Autodesk Inventor part; units mm, degrees
ref_plane "YZ Plane" through (0, 0, 0) normal (1, 0, 0) x (0, 1, 0)
ref_plane "XZ Plane" through (0, 0, 0) normal (0, 1, 0) x (-1, 0, 0)
ref_plane "XY Plane" through (0, 0, 0) normal (0, 0, 1) x (1, 0, 0)
sketch "Sketch1" plane through (0, 0, 0) normal (0, 1, 0) x (-1, 0, 0)
  line L0 (0, 0) -> (73.025, 0)
  line L1 (0, 0) -> (0, 73.025)
  line L2 (0, 73.025) -> (73.025, 0)
  line L3 (12.7, 0) -> (12.7, 60.325) construction
  line L4 (0, 12.7) -> (60.325, 12.7) construction
  circle A0 centre (12.7, 34.925) radius 3.302
  circle A1 centre (34.925, 12.7) radius 3.302
  circle A2 centre (50.8, 12.7) radius 3.302
  circle A3 centre (12.7, 50.8) radius 3.302
  circle A4 centre (12.7, 12.7) radius 3.302
  line L5 (0, 34.925) -> (38.1, 34.925) construction
  line L6 (34.925, 38.1) -> (34.925, 0) construction
  dimension "d0" = 73.025
  dimension "d1" = 73.025
  dimension "d2" = 12.7
  dimension "d3" = 12.7
  dimension "d4" = 6.604
  dimension "d5" = 6.604
  dimension "d6" = 6.604
  dimension "d7" = 6.604
  dimension "d8" = 15.875
  dimension "d9" = 15.875
  dimension "d10" = 6.604
  dimension "d14" = 34.925
  dimension "d15" = 34.925
extrude "Extrusion1" add sketch "Sketch1" along normal blind 3.175
fillet "Fillet1" radius 6.35 2 edges at (0, 1.5875, 73.025) (-73.025, 1.5875, 0)
equation "\"d0\" = d1"
equation "\"d2\" = d3"
equation "\"d4\" = d7"
equation "\"d5\" = d7"
equation "\"d6\" = d7"
equation "\"d9\" = d8"
equation "\"d10\" = d7"
equation "\"d15\" = d14"
properties part number "Chassis Corner Plate V1.500" material "Aluminum 6061"
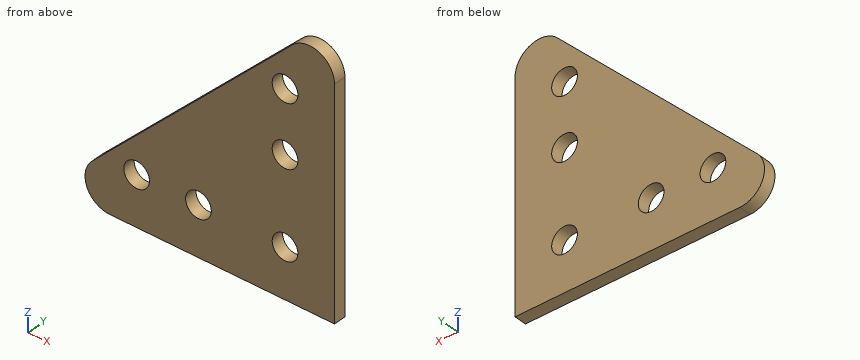
Could you check a few things on this model? Use its own coordinates, in mm. Coordinates: 2 decimals unless noted, no trailing zeros. Order: outer loops, then holes, each group sorted by start corner. A loop starts at its lowest first (then second) coordinate and runs counter-clockwise, first axis right, second up.
Q1. Suppose I cut it at A-A on z = 50.8. Please give me the cut outline in (x, y) (3 decimals).
Q2. Suppose I cut it at B-B on x = -12.7. Please give me the cut outline in (y, z) (3 decimals).
Q3. Suppose I cut it at C-C on y = 2.4. Please give me the cut outline in (x, z) (3 decimals), and give its area (3 significant figures).
Q4. Please list where these lines run through material, in increasing order: L1, parallel to Z at x = -12.7, y = 2.4 (3 decimals); L2, parallel to Z at x = -50.8, y = 1.3 (3 decimals); L3, parallel to X at y = 2.7, z = 11 (3 decimals).
Q5. Suppose I cut it at D-D on z = 12.7. Please give me the cut outline in (x, y) (3 decimals).
Answer:
1. outline: (-22.225, 0) - (-16.002, 0) - (-16.002, 3.175) - (-22.225, 3.175) - close; (-9.398, 0) - (0, 0) - (0, 3.175) - (-9.398, 3.175) - close
2. outline: (0, 0) - (3.175, 0) - (3.175, 9.398) - (0, 9.398) - close; (0, 16.002) - (3.175, 16.002) - (3.175, 31.623) - (0, 31.623) - close; (0, 38.227) - (3.175, 38.227) - (3.175, 47.498) - (0, 47.498) - close; (0, 54.102) - (3.175, 54.102) - (3.175, 60.325) - (0, 60.325) - close
3. outline: (-62.185, 10.84) arc R6.35 ccw to (-57.695, 0) - (0, 0) - (0, 57.695) arc R6.35 ccw to (-10.84, 62.185) - close; hole circle Ø6.604 at (-50.8, 12.7); hole circle Ø6.604 at (-34.925, 12.7); hole circle Ø6.604 at (-12.7, 12.7); hole circle Ø6.604 at (-12.7, 34.925); hole circle Ø6.604 at (-12.7, 50.8)
3. area: 2,400 mm2
4. L1: z = 0 to 9.398, 16.002 to 31.623, 38.227 to 47.498, 54.102 to 60.325
4. L2: z = 0 to 9.398, 16.002 to 22.225
4. L3: x = -62.025 to -53.631, -47.969 to -37.756, -32.094 to -15.531, -9.869 to 0
5. outline: (-60.325, 0) - (-54.102, 0) - (-54.102, 3.175) - (-60.325, 3.175) - close; (-47.498, 0) - (-38.227, 0) - (-38.227, 3.175) - (-47.498, 3.175) - close; (-31.623, 0) - (-16.002, 0) - (-16.002, 3.175) - (-31.623, 3.175) - close; (-9.398, 0) - (0, 0) - (0, 3.175) - (-9.398, 3.175) - close
